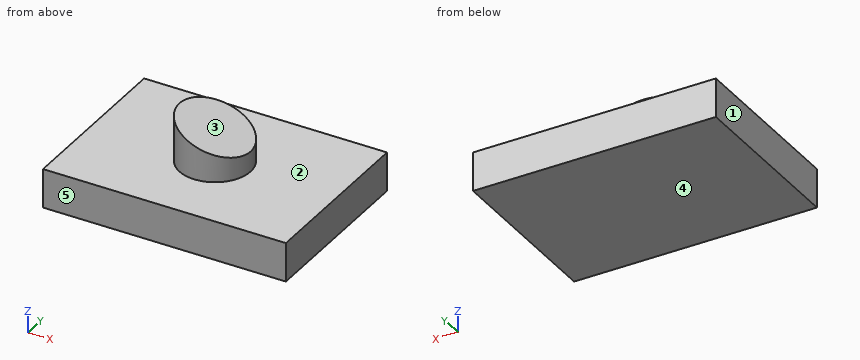
from build123d import *

# Parameters (mm, degrees)
F0_W     = 79.076722
F0_H     = 56.460418
F1_DEPTH = 12.7
F2_R     = 11.586166
F3_DEPTH = 23.368
F5_DEPTH = 20.828
F6_DEPTH = 37.338


with BuildPart() as f1:
    # F0 (on Top) → F1 (new body)
    with BuildSketch(Plane.XY):
        Rectangle(F0_W, F0_H)
    extrude(amount=F1_DEPTH)

    # F2 (on face) → F3 (join)
    with BuildSketch(Plane.XY.offset(12.7)):
        Circle(F2_R)
    extrude(amount=F3_DEPTH)

    # F4 (on Front) → F5 (cut)
    with BuildSketch(Plane.XZ):
        Polygon((-16.648348, 45.342267), (-16.648348, 30.036526), (12.731089, 18.900771), (12.731089, 45.342267), align=None)
    extrude(amount=-F5_DEPTH, mode=Mode.SUBTRACT)

    # F4 (on Front) → F6 (cut)
    with BuildSketch(Plane.XZ):
        Polygon((-16.648348, 45.342267), (-16.648348, 30.036526), (12.731089, 18.900771), (12.731089, 45.342267), align=None)
    extrude(amount=F6_DEPTH, mode=Mode.SUBTRACT)


solid = f1.part
For this review, take the finished solid that the model builds, in its own axes (mm). Face numbers are marked on the shaded views. A direction names the side the tool comes from. Coordinates: 2 decimals unless noted, no trailing zeros. Loops run counter-clockwise (first coordinate to the right, second up) from the corner with the lowest first, then second, coordinate; pieces in that order, holes last. Notation, with made-up numbers: (6.25, 60.5) - (30.25, 60.5) arc R17 cw to (30.25, 66.5) - close; hole circle Ø10 at (43.5, 21.25). An arc over 180 degrees is marked (long way). Use a Markdown table: item, result. Add a question column.
Item 1: We need section C-C (z = 17.5). Give the boundary of the cut face in (x, y).
Item 2: Insertion check: pin 1 Ø12 at (x, y) = (-5.5, -16.5) entering from +Z; pin 2 Ø3 at (x, y) = (-17.5, -10.5) entering from +Z. Each pin has a flat end and moves straight along its axis. Give the tip position at first contact, or say it passes through.
Item 3: We need section B-B (x = 0.5). Give the boundary of the cut face in (y, z), and give its area (3 significant figures).
Item 4: Mouldability with a two-part tool opening along Z and no side actions: class the marked faces 3, 4 and 5 as pulls with the +Z half, pulls with the -Z half, needs draft (parallel to the pull), parting line crosses it, or undercut.
Item 5: We need section A-A (y = 0). Give the boundary of the cut face in (x, z).
Item 6: Tool access review of the marked faces 1 and 2: name each direction out of +Z, -Z, +X, -X, +Y, -Y from which nothing blocks a thin tool from reaching the whole face with its end or side.
Item 7: For line 1 (Z direction, x = -32, y = 23.5); line 2 (Y direction, x = -6, z = 15.25); line 3 (X direction, y = 4.5, z = 17), list the stretches that pass through material, from the lowest coordinate up.
Item 8: We need section D-D (x = -27). Give the boundary of the cut face in (y, z), and give its area (3 significant figures).
Results list:
| question | item | result |
|---|---|---|
| 1 | outline | circle Ø23.17 at (0, 0) |
| 2 | pin 1 | stops at z = 25.55 |
| 2 | pin 2 | stops at z = 12.7 |
| 3 | outline | (-28.23, 0) - (28.23, 0) - (28.23, 12.7) - (11.58, 12.7) - (11.58, 23.54) - (-11.58, 23.54) - (-11.58, 12.7) - (-28.23, 12.7) - close |
| 3 | area | 968 mm^2 |
| 4 | face 3 | pulls with the +Z half |
| 4 | face 4 | pulls with the -Z half |
| 4 | face 5 | needs draft |
| 5 | outline | (-39.54, 0) - (39.54, 0) - (39.54, 12.7) - (11.59, 12.7) - (11.59, 19.33) - (-11.59, 28.12) - (-11.59, 12.7) - (-39.54, 12.7) - close |
| 6 | face 1 | +Z, -Z, -X, +Y, -Y |
| 6 | face 2 | +Z |
| 7 | line 1 | z = 0 to 12.7 |
| 7 | line 2 | y = -9.91 to 9.91 |
| 7 | line 3 | x = -10.68 to 10.68 |
| 8 | outline | (-28.23, 0) - (28.23, 0) - (28.23, 12.7) - (-28.23, 12.7) - close |
| 8 | area | 717 mm^2 |
